from build123d import *

# Parameters (mm, degrees)
SKETCH1_R           = 2.75
BOSS_EXTRUDE1_DEPTH = 2
FILLET1_R           = 1


with BuildPart() as part:
    # Sketch1 → Boss-Extrude1 (new body, symmetric)
    with BuildSketch(Plane.XY):
        Polygon((0, 0), (0, 18), (20, 58), (38, 58), (58, 18), (58, 0), align=None)
        with Locations((9, 9)):
            Circle(SKETCH1_R, mode=Mode.SUBTRACT)
        with Locations((29, 9)):
            Circle(SKETCH1_R, mode=Mode.SUBTRACT)
        with Locations((49, 9)):
            Circle(SKETCH1_R, mode=Mode.SUBTRACT)
        with Locations((29, 29)):
            Circle(SKETCH1_R, mode=Mode.SUBTRACT)
        with Locations((29, 49)):
            Circle(SKETCH1_R, mode=Mode.SUBTRACT)
    extrude(amount=BOSS_EXTRUDE1_DEPTH, both=True)

    # Fillet1
    fillet1_edges = [part.edges().sort_by_distance(p)[0] for p in [
        (48, 38, 2),
        (0, 0, 0),
        (0, 18, 0),
        (20, 58, 0),
        (38, 58, 0),
        (58, 18, 0),
        (58, 0, 0),
        (29, 58, 2),
        (10, 38, 2),
        (0, 9, 2),
        (29, 0, 2),
        (58, 9, 2),
    ]]
    fillet(fillet1_edges, radius=FILLET1_R)


solid = part.part
Could you check a few things on this model? Use its own coordinates, in mm. Coordinates: 2 decimals unless noted, no trailing zeros. Loops run counter-clockwise (first coordinate to the right, second up) from the corner with the lowest first, then second, coordinate; pieces in that order, holes last.
1. Imagine slicing it at B-B (z = 0.25). Please give me the cut outline in (x, y), and give its area (3 significant figures).
2. I need wall thicknesses on L1, parallel to Y at x = 29, z = 0.9; L2, parallel to X at y = 8, z = 0.4; L3, parallel to X at y = 27, z = -1.5. Which ranges of each line are inside material? Lowest first, please.
3. We'd pull the mould along Y, two halves only. Please class faces 1 (the face through (29, 0, 0)), 2 (the face through (26.253, 29.121, -0.028)), 3 (the face through (58, 9, 0)): released by +Y, released by -Y, zero draft, split by the parting line, or undercut.
4. Imagine slicing it at A-A (y = 9). Please give me the cut outline in (x, z), and give its area (3 significant figures).
Computed values:
1. outline: (0, 1) arc R1 ccw to (1, 0) - (57, 0) arc R1 ccw to (58, 1) - (58, 17.76) arc R1 ccw to (57.89, 18.21) - (38.28, 57.45) arc R1 ccw to (37.38, 58) - (20.62, 58) arc R1 ccw to (19.72, 57.45) - (0.11, 18.21) arc R1 ccw to (0, 17.76) - close; hole circle Ø5.5 at (9, 9); hole circle Ø5.5 at (29, 9); hole circle Ø5.5 at (29, 29); hole circle Ø5.5 at (29, 49); hole circle Ø5.5 at (49, 9)
1. area: 2,440 mm2
2. L1: y = 0 to 6.25, 11.75 to 26.25, 31.75 to 46.25, 51.75 to 58
2. L2: x = 0 to 6.44, 11.56 to 26.44, 31.56 to 46.44, 51.56 to 58
2. L3: x = 4.5 to 27.11, 30.89 to 53.5
3. face 1: released by -Y
3. face 2: undercut
3. face 3: zero draft
4. outline: (0, -2) - (6.25, -2) - (6.25, 2) - (1, 2) arc R1 ccw to (0, 1) - close; (11.75, -2) - (26.25, -2) - (26.25, 2) - (11.75, 2) - close; (31.75, -2) - (46.25, -2) - (46.25, 2) - (31.75, 2) - close; (51.75, -2) - (58, -2) - (58, 1) arc R1 ccw to (57, 2) - (51.75, 2) - close
4. area: 166 mm2
